Build history of the part. All positions in model axes, mm. A direction names the side the tool comes from. Give positions to 0.01 mm unless a question says otherwise; leave off trailing zeros. Loops run counter-clockwise (first coordinate to the right, second up) from the corner with the lowest first, then second, coordinate; pieces in that order, holes last. Notation, with made-up numbers: (52, -5) - (69, -5) arc R17 ccw to (69, 11) - close; hole circle Ø7 at (53.25, 23). An arc over 180 degrees is marked (long way). Return JSON: item names as keys, results as strings. Group by question number.
1) Slice it at C-C (x = 13). List the corners of the cut face in (y, z), and give its area (3 significant figures).
2) Drop flat-ended pins along their axis: pin 1 (13 mm diameter, centred on y = -10.5, z = 119, fed in from -X); pin 2 (17.5 mm diameter, centred on x = 47, y = 14, fed in from -Z); pin 3 (19 mm diameter, centred on x = 36, y = 42.5, fed in from +Z); pin 4 (12 mm diameter, centred on x = 40.5, z = -24.5, fed in from -Y). Give the stop position or say it passes through.
3) Drill centre lines: probe 1 along Y at (x, z) = (39, 81); probe 2 along X at (y, z) = (-102.5, 60.5); probe 3 along Z at (x, y) = (39.5, -67). Where is each one in solid material? Low to high. Write a range as from..to.
4) Slice it at B-B (z = -4). List the corners of the cut face in (x, y), and give its area (3 significant figures).
5) Mould opens along Y. For faces 4 (the face through (24, -161.866, 13)), 5 (the face through (5.08, -7, -12)), 6 (the face through (36.48, 140.26, -11.98)), 7 (the face through (28, -156.786, 10)) say: released by +Y, released by -Y, zero draft, split by the parting line, or undercut.
6) 3-axis set-ups, long thin cutter, end or side, ignore diameter. For faces 1 (the face through (35, -14, 85.568)), 2 (the face through (50, -21.308, 109)), 3 (the face through (50, 4.482, 109)): which of +Z, -Z, +X, -X, +Y, -Y reach the whole face in a straight line?
7) Slice it at A-A (y = 112). List the corners of the cut face in (x, z), and give its area (3 significant figures).
8) Slice it at D-D (z = 98.5). List the corners of the cut face in (x, y).
```python
from build123d import *

# Parameters (mm, degrees)
F0_W      = 304.7006875277
F0_H      = 202.9495164752
F1_DEPTH  = 63.5
F2_T      = -5.08
F3_DEPTH  = 25.4
F4_DEPTH  = 25.4
F7_DEPTH  = 123.952
F9_DEPTH  = 25.4
F10_W     = 5.08
F10_H     = 197.8695164752
F11_DEPTH = 0.508
F12_W     = 25.8265564442
F12_H     = 25.7899604912
F13_DEPTH = 38.1


with BuildPart() as f1:
    # F0 (on Right) → F1 (new body)
    with BuildSketch(Plane.YZ):
        with Locations((-9.5159932971, -10.8270607889)):
            Rectangle(F0_W, F0_H)
    extrude(amount=F1_DEPTH)

    # F2
    f2_openings = [f1.faces().sort_by_distance(p)[0] for p in [
        (63.5, -9.515993, -10.827061),
    ]]
    offset(amount=F2_T, openings=f2_openings)

    # F3 (cut): a face of the model
    f3_faces = [f1.faces().sort_by_distance(p)[0] for p in [
        (31.75, -9.5159932971, -112.3018190265),
    ]]
    extrude(f3_faces, amount=-F3_DEPTH, mode=Mode.SUBTRACT)

    # F4 (add): a face of the model
    f4_faces = [f1.faces().sort_by_distance(p)[0] for p in [
        (3.1124710277, -9.5159932971, -86.9018190265),
    ]]
    extrude(f4_faces, amount=F4_DEPTH)

    # F6 (on face) → F7 (cut)
    with BuildSketch(Plane.XZ.offset(-137.7543504667)):
        Polygon((63.5, -112.3018190265), (63.5, 85.5676974487), (8.6876470596, -112.3018190265), align=None)
    extrude(amount=-F7_DEPTH, mode=Mode.SUBTRACT)

    # F8 (on face) → F9 (cut)
    with BuildSketch(Plane(origin=(0, -156.7863370609, 0), x_dir=(-1, 0, 0), z_dir=(0, 1, 0))):
        Polygon((-8.4076998755, -112.942405045), (-63.1341859698, 84.8678573966), (-63.1341859698, -112.942405045), align=None)
    extrude(amount=-F9_DEPTH, mode=Mode.SUBTRACT)

    # F10 (on face) → F11 (cut)
    with BuildSketch(Plane.YZ.offset(63.5)):
        with Locations((-159.3263370609, -13.3670607889)):
            Rectangle(F10_W, F10_H)
    extrude(amount=-F11_DEPTH, mode=Mode.SUBTRACT)

    # F12 (on face) → F13 (join)
    with BuildSketch(Plane.XY.offset(90.6476974487)):
        with Locations((50.5867217779, -8.4131233307)):
            Rectangle(F12_W, F12_H)
    extrude(amount=F13_DEPTH)


solid = f1.part
```
Results:
{
 "1": {"outline": "(-161.87, -96.34) - (-156.79, -96.34) - (-156.79, 85.57) - (137.75, 85.57) - (137.75, -96.73) - (142.83, -96.73) - (142.83, 90.65) - (-161.87, 90.65) - close", "area": "3,400 mm2"},
 "2": {"pin 1": "x = 37.67", "pin 2": "z = 85.57", "pin 3": "z = 90.65", "pin 4": "through"},
 "3": {"probe 1": "-161.87..-156.79, 137.75..142.83", "probe 2": "0..5.08", "probe 3": "85.57..90.65"},
 "4": {"outline": "(0, -161.87) - (38.55, -161.87) - (38.55, -156.79) - (5.08, -156.79) - (5.08, 137.75) - (38.69, 137.75) - (38.69, 142.83) - (0, 142.83) - close", "area": "1,890 mm2"},
 "5": {"face 4": "released by -Y", "face 5": "undercut", "face 6": "zero draft", "face 7": "undercut"},
 "6": {"face 1": "-Z, +X", "face 2": "+Z, +X, -X, -Y", "face 3": "+Z, +X, -X, +Y"},
 "7": {"outline": "(0, -112.3) - (5.08, -112.3) - (5.08, 85.57) - (63.5, 85.57) - (63.5, 90.65) - (0, 90.65) - close", "area": "1,330 mm2"},
 "8": {"outline": "(37.67, -21.31) - (63.5, -21.31) - (63.5, 4.48) - (37.67, 4.48) - close"}
}
